Answer from the drawing. Dimensions are ordinates in mm from the lowest x, y and z of the part. A direction names the side the tool comes from. Round coordinates to 2 decimals unless told otherwise and drop trailing zeros. Loops run counter-clockwise (first coordinate to the right, second up) from the corner with the lowest first, then second, coordinate; pieces in that order, holes last. Notation, with made-up numbers: M 77,50.5 L 113,50.5 A18 ccw 113,64.5 Z; hole C 89,61 d2. An arc over 180 degrees is marked long. One line per item, written item: value.
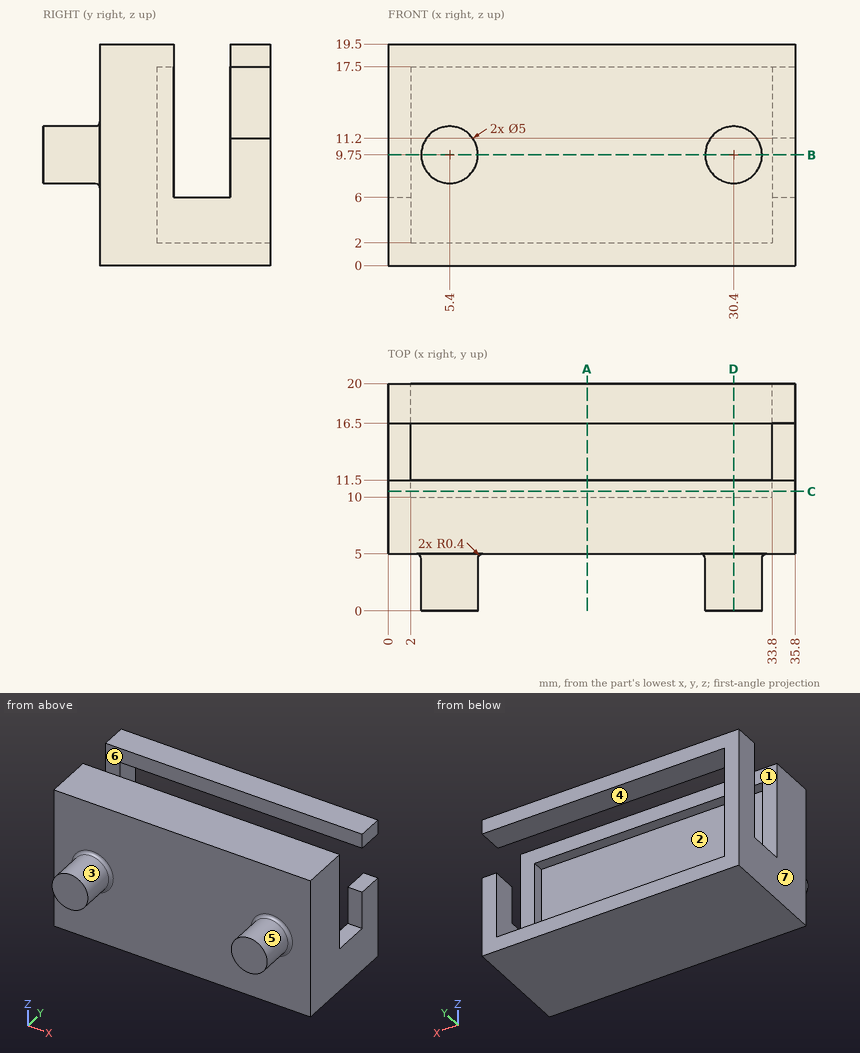
1) Find section A-A (x = 17.5). Give the vertices of the cut face in (y, z).
Check values:
outline: M 5,0 L 20,0 L 20,2 L 10,2 L 10,17.5 L 11.5,17.5 L 11.5,19.5 L 5,19.5 Z; M 16.5,17.5 L 20,17.5 L 20,19.5 L 16.5,19.5 Z
2) The mould has two halves that part along X. Classify the marked faces 5, 6 and 7: +X half, -X half, draft (parallel to the pull), parting line (faces both ways), or undercut.
Check values:
face 5: undercut
face 6: draft
face 7: -X half
3) Find section D-D (x = 30.4). Give the vertices of the cut face in (y, z), then the cut area to 3 significant figures.
Check values:
outline: M 0,7.25 L 4.6,7.25 A0.4 cw 5,6.85 L 5,0 L 20,0 L 20,2 L 10,2 L 10,17.5 L 11.5,17.5 L 11.5,19.5 L 5,19.5 L 5,12.65 A0.4 cw 4.6,12.25 L 0,12.25 Z; M 16.5,17.5 L 20,17.5 L 20,19.5 L 16.5,19.5 Z
area: 153 mm2
4) Each of these flat-tipped pins is pushed along its axis until it touches: pin 1 (1.6 mm diameter, centred on x = 0.5, y = 13.5, fed in from +Z); pin 2 (4 mm diameter, centred on x = 23, z = 10, fed in from -Y); pin 3 (4.5 mm diameter, centred on x = 10.5, z = 11.5, fed in from +Y). Where does it stop, or does it pass through?
Check values:
pin 1: z = 6
pin 2: y = 5
pin 3: y = 10
5) For the marked faces 1, 2, 3 and 4, determine the directions among +Z, -Z, +X, -X, +Y, -Y from which every point of the face is accessible in a straight line to the end or side of a thin tool.
Check values:
face 1: +Z, +X, -X
face 2: +Y
face 3: -Y
face 4: +X, +Y
6) Find section C-C (y = 10.5). Give the vertices of the cut face in (x, z), then the cut area to 3 significant figures.
Check values:
outline: M 0,0 L 35.8,0 L 35.8,19.5 L 0,19.5 Z; hole M 2,2 L 33.8,2 L 33.8,17.5 L 2,17.5 Z
area: 205 mm2
7) Find section B-B (z = 9.75). Give the vertices of the cut face in (x, y).
Check values:
outline: M 0,5 L 2.5,5 A0.4 cw 2.9,4.6 L 2.9,0 L 7.9,0 L 7.9,4.6 A0.4 cw 8.3,5 L 27.5,5 A0.4 cw 27.9,4.6 L 27.9,0 L 32.9,0 L 32.9,4.6 A0.4 cw 33.3,5 L 35.8,5 L 35.8,11.5 L 33.8,11.5 L 33.8,10 L 2,10 L 2,11.5 L 0,11.5 Z; M 0,16.5 L 2,16.5 L 2,20 L 0,20 Z; M 33.8,16.5 L 35.8,16.5 L 35.8,20 L 33.8,20 Z
8) Find the intervals of material crossed by probe 1 along X at (y, z) = (18.75, 6); probe 2 along Z at (x, y) = (30, 19); probe 3 along Y at (x, z) = (32, 9), in increasing order. Write a range as from..to.
Check values:
probe 1: 0..2, 33.8..35.8
probe 2: 0..2, 17.5..19.5
probe 3: 0..10
